Design review of the part built by this model. Coordinates are the model's own, in mm. A direction names the side the tool comes from. Round coordinates to 2 decimals unless told otherwise and drop trailing zeros. Order: outer loops, then holes, each group sorted by start corner. A loop starts at its lowest first (then second) coordinate and runs counter-clockwise, first axis right, second up. Notation, with made-up numbers: (-4, 85) - (7, 85) arc R25 ccw to (7, 122) - close; hole circle Ø6 at (25, -27). An arc over 180 degrees is marked (long way). Write item = value, one per line.
from build123d import *

# Parameters (mm, degrees)
SKETCH1_R                   = 30.1625
SKETCH1_R_2                 = 12.7
SKETCH1_R_3                 = 4.7625
BOSS_EXTRUDE1_DEPTH         = 5
BOSS_EXTRUDE2_START         = 6.5
SKETCH1_3_R                 = 12.7
SKETCH1_3_R_2               = 4.7625
BOSS_EXTRUDE2_DEPTH         = 6.5
F_10_CLEARANCE_HOLE1_D      = 4.9784
TAP_DRILL_FOR_M3X0_5_TAP1_D = 2.5
FILLET1_R                   = 0.79375


with BuildPart() as part:
    # Sketch1 → Boss-Extrude1 (new body)
    # profile 1 of 2: a face of its own
    with BuildSketch(Plane(origin=(0, 0, 0), x_dir=(1, 0, 0), z_dir=(0, 1, 0))):
        with Locations(Location((0, 0, 0), (0, 0, 270))):
            Circle(SKETCH1_R)
        Circle(SKETCH1_R_2, mode=Mode.SUBTRACT)
    # profile 2 of 2: a face of its own
    with BuildSketch(Plane(origin=(0, 0, 0), x_dir=(1, 0, 0), z_dir=(0, 1, 0))):
        Circle(SKETCH1_R_2)
        with Locations(Location((0, 0, 0), (0, 0, 270))):
            Circle(SKETCH1_R_3, mode=Mode.SUBTRACT)
    extrude(amount=-BOSS_EXTRUDE1_DEPTH)

    # Sketch1<3> → Boss-Extrude2 (add)
    with BuildSketch(Plane(origin=(0, 0, 0), x_dir=(1, 0, 0), z_dir=(0, 1, 0)).offset(BOSS_EXTRUDE2_START)):
        with Locations(Location((0, 0, 0), (0, 0, 90))):
            Circle(SKETCH1_3_R)
        with Locations(Location((0, 0, 0), (0, 0, 270))):
            Circle(SKETCH1_3_R_2, mode=Mode.SUBTRACT)
    extrude(amount=-BOSS_EXTRUDE2_DEPTH)

    # #10 Clearance Hole1 (through all)
    with Locations(Plane(origin=(0, 0, -23.8125), x_dir=(0, 0, 1), z_dir=(0, 1, 0))):
        with Locations((0, 0), (11.90625, 20.622229928), (35.71875, 20.622229928), (11.90625, -20.622229928), (35.71875, -20.622229928), (47.625, 0)):
            Hole(F_10_CLEARANCE_HOLE1_D / 2)

    # Tap Drill for M3x0.5 Tap1 (through all)
    with Locations(Plane(origin=(0, 3.25, 12.7), x_dir=(1, 0, 0), z_dir=(0, 0, 1))):
        with Locations((0, 0)):
            Hole(TAP_DRILL_FOR_M3X0_5_TAP1_D / 2)

    # Fillet1
    fillet1_edges = [part.edges().sort_by_distance(p)[0] for p in [
        (0, 6.5, 12.7),
        (0, 0, -30.1625),
    ]]
    fillet(fillet1_edges, radius=FILLET1_R)


solid = part.part
Item 1: Insertion check: P1, Ø3, axis at x = -20.62, z = -11.91, coming from the +Y side (3 decimals); P2, Ø6, axis at y = -2, z = 16, coming from the +X side; P3, Ø1.5, axis at y = -2.5, z = 18, coming from the -X side; P4, Ø3, axis at x = 0, y = 3.25, coming from the +Z side. Each pin has a flat end and moves straight along its axis. Give the tip position at first contact, or say it passes through.
Data:
P1 = through
P2 = 27.22
P3 = -24.74
P4 = 12.7
Item 2: The part is to be moulded in two halves that separate along X. For faces 1 (the face through (-22.831, -2.535, -13.055)), 2 (the face through (1.326, -2.867, -30.133)), 3 (the face through (0, 0, -13)), 4 (the face through (0.16, 4.49, -8.7)), say which applies: +X half, -X half, draft (parallel to the pull), parting line (faces both ways), or undercut.
Data:
face_1 = undercut
face_2 = parting line
face_3 = draft
face_4 = undercut
Item 3: For line 1 along Z through (x, y) = (0.5, -1.5); line 2 along X through (y, z) = (-0.25, 13); line 3 along X through (y, z) = (-2, -13), list the stretches that pass through material, from the lowest coordinate up. Write a range as [from, to].
Data:
line_1 = [-30.16, -26.25], [-21.37, -4.74], [4.74, 21.37], [26.25, 30.16]
line_2 = [-26.98, -22.86], [-18.39, 18.39], [22.86, 26.98]
line_3 = [-27.22, -22.86], [-18.39, 18.39], [22.86, 27.22]
Item 4: For faces 5 (the face through (-22.83, -2.53, 10.76)), 6 (the face through (-3.815, 2.893, -12.114)), list the 3-axis set-ups (+Z, -Z, +X, -X, +Y, -Y) from which the entire face can be reached by the end or side of a thin tool; tool diameter is ignored.
Data:
face_5 = +Y, -Y
face_6 = +Y
Item 5: Take a section at D-D, the plane y = -2.25. State the section outline as (x, z) points (1 decimal).
Data:
outline = circle Ø60.3 at (0, 0); hole circle Ø5 at (-20.6, -11.9); hole circle Ø5 at (-20.6, 11.9); hole circle Ø9.5 at (0, 0); hole circle Ø5 at (0, -23.8); hole circle Ø5 at (0, 23.8); hole circle Ø5 at (20.6, -11.9); hole circle Ø5 at (20.6, 11.9)
Item 6: Take a section at B-B, the plane z = 0. State the section outline as (x, y) points, and give its area (3 significant figures).
Data:
outline = (-30.16, -5) - (-4.76, -5) - (-4.76, 6.5) - (-11.91, 6.5) arc R0.79 ccw to (-12.7, 5.71) - (-12.7, 0) - (-29.37, 0) arc R0.79 ccw to (-30.16, -0.79) - close; (4.76, -5) - (30.16, -5) - (30.16, -0.79) arc R0.79 ccw to (29.37, 0) - (12.7, 0) - (12.7, 5.71) arc R0.79 ccw to (11.91, 6.5) - (4.76, 6.5) - close
area = 357 mm2
Item 7: Take a section at A-A, the plane x = 0. Count the separate pieces of the cut face and the enclosed holes in it, and give its area (3 significant figures).
Data:
separate_pieces = 6
enclosed_holes = 0
area = 267 mm2
